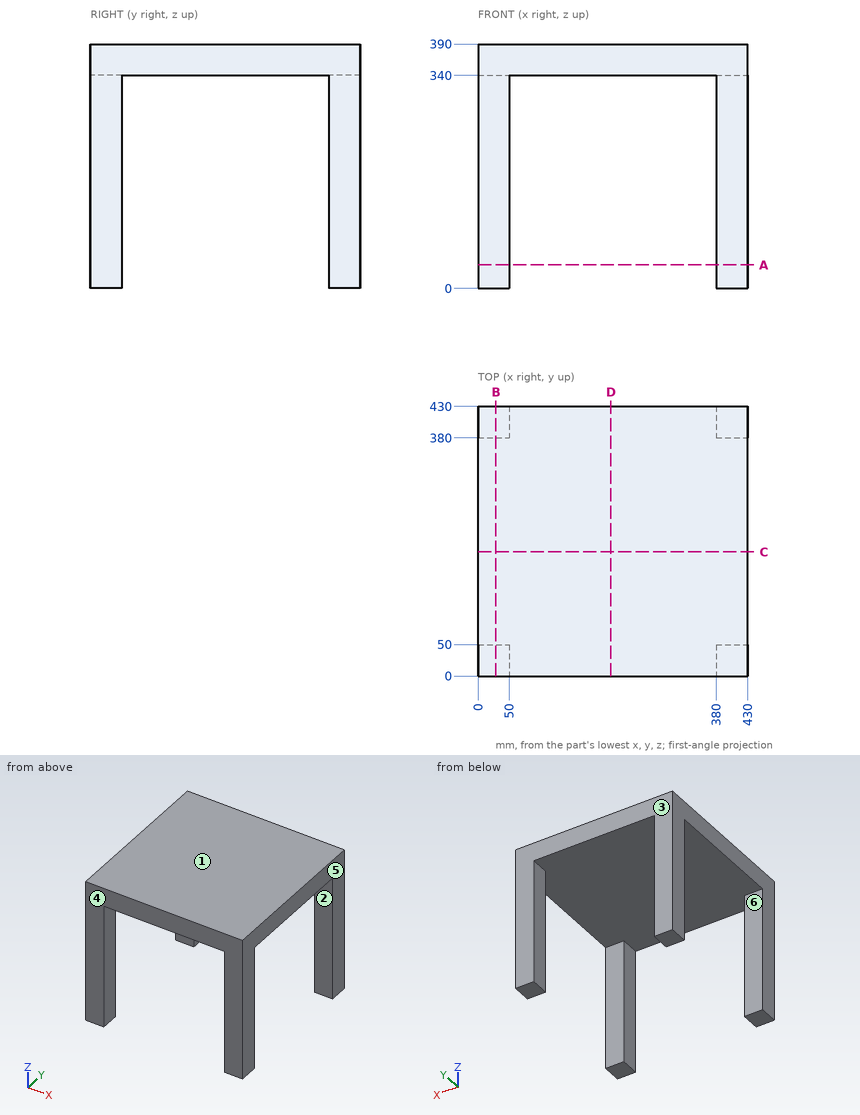
The figure shows three views and two pictorial views of one solid part (mm, origin at its lowest corner). Answer the questions. A direction names the side the tool comes from. Give positions to 0.01 mm unless a question says otherwise; leave off trailing zeros. Write each loop counter-clockwise with the first axis right and the second up, starting at its lowest first coordinate (ties: lowest second). Pieces come first, ordered by that corner, then holes.
Q1. Straight lines are drawn through the part: L1, parallel to Y at x = 412.5, z = 54; L2, parallel to Z at x = 182.5, y = 25.5. For each, find the intervals that lie inside material, in ascending order.
Answer:
L1: y = 0 to 50, 380 to 430
L2: z = 340 to 390
Q2. The part is cut by section A-A on z = 37.5. Give the vertices of the cut face in (x, y), and give its area (3 significant figures).
Answer:
outline: (0, 0) - (50, 0) - (50, 50) - (0, 50) - close; (0, 380) - (50, 380) - (50, 430) - (0, 430) - close; (380, 0) - (430, 0) - (430, 50) - (380, 50) - close; (380, 380) - (430, 380) - (430, 430) - (380, 430) - close
area: 10,000 mm2
Q3. The part is cut by section B-B on x = 28.5. Give the vertices of the cut face in (y, z), and give its area (3 significant figures).
Answer:
outline: (0, 0) - (50, 0) - (50, 340) - (380, 340) - (380, 0) - (430, 0) - (430, 390) - (0, 390) - close
area: 55,500 mm2
Q4. The part is cut by section C-C on y = 198. Give the vertices of the cut face in (x, z).
Answer:
outline: (0, 340) - (430, 340) - (430, 390) - (0, 390) - close
Q5. A tool of negligible diameter and unlimited length cuts with its end or side. For the marked faces 5 and 6, from which of +Z, -Z, +X, -X, +Y, -Y can it reach the whole face along a straight path? Write none if from no direction.
Answer:
face 5: +Z, -Z, +X, +Y, -Y
face 6: -Z, +X, -X
Q6. For a pull along Y with two mould halves and no side action, classify the marked faces 1, 2, 3 and 4 as released by +Y, released by -Y, zero draft, split by the parting line, or undercut.
Answer:
face 1: zero draft
face 2: undercut
face 3: released by +Y
face 4: released by -Y
